from build123d import *

# Parameters (mm, degrees)
SKETCH1_W                = 134
SKETCH1_H                = 134
SKETCH1_W_2              = 20
SKETCH1_H_2              = 13
BOSS_EXTRUDE1_DEPTH      = 1.5
BOSS_EXTRUDE2_DEPTH      = 45
SKETCH2_R                = 1.35
CUT_EXTRUDE1_DEPTH       = 137.5
SKETCH3_W                = 53.4
SKETCH3_H                = 43.5
CUT_EXTRUDE2_DEPTH       = 137.5
SKETCH4_W                = 140
SKETCH4_H                = 5
CUT_EXTRUDE3_DEPTH       = 1.5
SKETCH5_W                = 30
SKETCH5_H                = 43.5
CUT_EXTRUDE4_DEPTH       = 137.5
CUT_EXTRUDE5_DEPTH       = 10
BOSS_EXTRUDE3_DEPTH      = 1.5
BOSS_EXTRUDE4_DEPTH      = 1
BOSS_EXTRUDE5_DEPTH      = 30
BOSS_EXTRUDE5_DEPTH_BACK = 1.5
CUT_EXTRUDE6_DEPTH       = 137.5
SKETCH11_W               = 5
SKETCH11_H               = 40
CUT_EXTRUDE7_DEPTH       = 1.5
BOSS_EXTRUDE6_DEPTH      = 1.5


with BuildPart() as part:
    # Sketch1 → Boss-Extrude1 (new body)
    with BuildSketch(Plane(origin=(0, 0, 0), x_dir=(1, 0, 0), z_dir=(0, 1, 0))):
        Rectangle(SKETCH1_W, SKETCH1_H)
        Rectangle(SKETCH1_W_2, SKETCH1_H_2, mode=Mode.SUBTRACT)
        Polygon((-67, 67), (-67.25, 67.25), (-67.25, -67.25), (67.25, -67.25), (67.25, 67.25), (67, 67), (67, -67), (-67, -67), align=None)
    extrude(amount=BOSS_EXTRUDE1_DEPTH)

    # Sketch1<3> → Boss-Extrude2 (add)
    with BuildSketch(Plane(origin=(0, 0, 0), x_dir=(1, 0, 0), z_dir=(0, 1, 0))):
        Polygon((-67.25, -67.25), (-67.25, 67.25), (-68.75, 68.75), (-68.75, -68.75), (68.75, -68.75), (68.75, 68.75), (67.25, 67.25), (67.25, -67.25), align=None)
    extrude(amount=BOSS_EXTRUDE2_DEPTH)

    # Sketch2 → Cut-Extrude1 (cut)
    with BuildSketch(Plane.ZY.offset(68.75)):
        with Locations((10.85, 42)):
            Circle(SKETCH2_R)
        with Locations((-29.15, 42)):
            Circle(SKETCH2_R)
    extrude(amount=-CUT_EXTRUDE1_DEPTH, mode=Mode.SUBTRACT)

    # Sketch3 → Cut-Extrude2 (cut)
    with BuildSketch(Plane.ZY.offset(68.75)):
        with Locations((40.55, 23.25)):
            Rectangle(SKETCH3_W, SKETCH3_H)
    extrude(amount=-CUT_EXTRUDE2_DEPTH, mode=Mode.SUBTRACT)

    # Sketch4 → Cut-Extrude3 (cut)
    with BuildSketch(Plane.XY.offset(68.75)):
        with Locations((0, 42.5)):
            Rectangle(SKETCH4_W, SKETCH4_H)
    extrude(amount=-CUT_EXTRUDE3_DEPTH, mode=Mode.SUBTRACT)

    # Sketch5 → Cut-Extrude4 (cut)
    with BuildSketch(Plane.ZY.offset(68.75)):
        with Locations((-53.75, 23.25)):
            Rectangle(SKETCH5_W, SKETCH5_H)
    extrude(amount=-CUT_EXTRUDE4_DEPTH, mode=Mode.SUBTRACT)

    # Sketch6 → Cut-Extrude5 (cut)
    with BuildSketch(Plane(origin=(0, 0, 0), x_dir=(-1, 0, 0), z_dir=(0, -1, 0))):
        Polygon((67, 67), (68.75, 67), (68.75, 68.75), align=None)
        Polygon((19.386551984, 67), (68.75, 38.5), (68.75, 67), (67, 67), align=None)
        Polygon((-68.75, 38.5), (-19.386551984, 67), (-67, 67), (-68.75, 67), align=None)
        Polygon((-68.75, 67), (-67, 67), (-68.75, 68.75), align=None)
    extrude(amount=-CUT_EXTRUDE5_DEPTH, mode=Mode.SUBTRACT)


with BuildPart() as body_2:
    # Sketch7 → Boss-Extrude3 (new body)
    with BuildSketch(Plane(origin=(-68.75, 0, 0), x_dir=(0, 0, -1), z_dir=(-1, 0, 0))):
        Polygon((49.15, -63.7), (38.75, -63.7), (38.75, -45), (19.55, -45), (19.55, -63.7), (4.15, -63.7), (4.15, -81.7), (49.15, -81.7), align=None)
    boss_extrude3 = extrude(amount=-BOSS_EXTRUDE3_DEPTH)


with BuildPart() as part_1:
    add(part.part)

    # Mirror6: Boss-Extrude3 across plane
    add(boss_extrude3.mirror(Plane(origin=(0, 0, 0), x_dir=(0, 0, 1), z_dir=(1, 0, 0))))


with BuildPart() as body_2_1:
    add(body_2.part)

    # Combine1: union part
    add(part_1.part)

    # Sketch8 → Boss-Extrude4 (add)
    with BuildSketch(Plane(origin=(0, 1.5, 0), x_dir=(1, 0, 0), z_dir=(0, 1, 0))):
        Polygon((-9.5, 37), (-9.5, 67), (-10.5, 67), (-10.5, 36), (0, 36), (0, 37), align=None)
        Polygon((10.5, 67), (9.5, 67), (9.5, 37), (0, 37), (0, 36), (10.5, 36), align=None)
    extrude(amount=BOSS_EXTRUDE4_DEPTH)

    # Sketch9 → Boss-Extrude5 (add, two sides)
    with BuildSketch(Plane(origin=(0, 1.5, 0), x_dir=(1, 0, 0), z_dir=(0, 1, 0))) as boss_extrude5_sk:
        Polygon((-19.386551984, 67), (-68.25, 38.5), (-68.753822513, 39.363807198), (-19.890374497, 67.863807198), align=None)
        Polygon((19.890374497, 67.863807198), (68.753822513, 39.363807198), (68.25, 38.5), (19.386551984, 67), align=None)
    extrude(amount=BOSS_EXTRUDE5_DEPTH)
    extrude(boss_extrude5_sk.sketch, amount=-BOSS_EXTRUDE5_DEPTH_BACK)

    # Sketch10 → Cut-Extrude6 (cut)
    with BuildSketch(Plane(origin=(68.75, 0, 0), x_dir=(0, 0, -1), z_dir=(1, 0, 0))):
        with BuildLine():
            Line((-13.85, 42), (-13.85, 45))
            Line((-13.85, 45), (-10.85, 45))
            ThreePointArc((-10.85, 45), (-12.971320344, 44.121320344), (-13.85, 42))
        make_face()
    extrude(amount=-CUT_EXTRUDE6_DEPTH, mode=Mode.SUBTRACT)

    # Sketch11 → Cut-Extrude7 (cut)
    with BuildSketch(Plane.XY.offset(68.75)):
        with Locations((66.25, 20)):
            Rectangle(SKETCH11_W, SKETCH11_H)
        with Locations((-66.25, 20)):
            Rectangle(SKETCH11_W, SKETCH11_H)
    extrude(amount=-CUT_EXTRUDE7_DEPTH, mode=Mode.SUBTRACT)


with BuildPart() as body_2_2:
    # Sketch12 → Boss-Extrude6 (new body)
    with BuildSketch(Plane(origin=(68.75, 0, 0), x_dir=(0, 0, -1), z_dir=(1, 0, 0))):
        Polygon((4.15, 63.7), (4.35, 45), (19.55, 45), (19.55, 63.7), align=None)
    extrude(amount=-BOSS_EXTRUDE6_DEPTH)


with BuildPart() as body_3:
    # Mirror8: mirrored copy
    add(body_2_2.part.mirror(Plane(origin=(0, 0, 0), x_dir=(0, 0, 1), z_dir=(1, 0, 0))))


with BuildPart() as body_2_2_1:
    add(body_2_2.part)

    # Combine2: union body 3, body 2
    add(body_3.part)
    add(body_2_1.part)


solid = body_2_2_1.part
Can you work these out from the model? Positions are in its coordinate system, mm. A direction names the side the tool comes from. Give positions to 0.01 mm unless a question says otherwise; leave off trailing zeros. Write each loop counter-clockwise with the first axis right and the second up, starting at its lowest first coordinate (ties: lowest second). Pieces come first, ordered by that corner, then holes. Notation, with made-up numbers: M 44.5,79 L 98.5,79 A31 cw 98.5,113 Z; hole C -15,24 d11. An arc over 180 degrees is marked long. Answer in a Markdown table with one row per item. Add a question column.
Item 1: Imagine slicing it at B-B, the plane y = 48. Write out the boundary of the cut face in (x, z), plus the area to 3 significant figures.
Item 2: Imagine slicing it at C-C, the plane y = 29. Write out the boundary of the cut face in (x, z), plus the area to 3 significant figures.
Item 3: Please list where these lines run through material, in increasing order: L1, parallel to X at y = 35.5, z = -35; L2, parallel to Y at x = -68, z = -29; L3, parallel to Y at x = -67.95, z = 10.85.
Item 4: For pin 1 Ø5 at (x, z) = (-44.5, 24.5) entering from +Y; pin 2 Ø1.1 at (x, y) = (3.5, 2) entering from -Z; pin 3 Ø19 at (y, z) = (25.5, -20) entering from -X, each with a flat end and sliding along its axis, tell me the tip position at first contact or that it passes through.
Item 5: On a 3-axis mill with a long thin cutter (end or side, diameter ignored), from which of +Z, -Z, +X, -X, +Y, -Y can I reach the whole of each face in a straight line? I mean faces 1 (the flat face through (-10, 2.5, -47)), 2 (the flat face through (67.25, 41, -17)), 3 (the flat face through (-1, 1.5, 14)). Say none if no direction works.
Item 6: Imagine slicing it at D-D, the plane x = 38. Write out the boundary of the cut face in (y, z), plus the area to 3 significant figures.
Item 7: We'd pull the mould along Z, two halves only. Please class faces 4 (the flat face through (-43.265, 16.29, -53.073)), 5 (the flat face through (-44.664, 15.97, -53.414)), 6 (the flat face through (0, 1.5, -52)): released by +Z, released by -Z, zero draft, split by the parting line, or undercut.
Item 8: Imagine slicing it at A-A, the plane z = 1. Write out the boundary of the cut face in (x, y).
Evaluation:
| question | item | result |
|---|---|---|
| 1 | outline | M -68.75,-38.75 L -67.25,-38.75 L -67.25,-4.32 L -68.75,-4.32 Z; M 67.25,-38.75 L 68.75,-38.75 L 68.75,-4.32 L 67.25,-4.32 Z |
| 1 | area | 103 mm² |
| 2 | outline | M -68.75,-39.36 L -19.89,-67.86 L -19.39,-67 L -67.82,-38.75 L -67.25,-38.75 L -67.25,13.85 L -68.75,13.85 L -68.75,-38.75 L -68.4,-38.75 Z; M -63.75,67.25 L 63.75,67.25 L 63.75,68.75 L -63.75,68.75 Z; M 19.39,-67 L 19.89,-67.86 L 68.75,-39.36 L 68.4,-38.75 L 68.75,-38.75 L 68.75,13.85 L 67.25,13.85 L 67.25,-38.75 L 67.82,-38.75 Z |
| 2 | area | 462 mm² |
| 3 | L1 | x = -68.75 to -67.25, 67.25 to 68.75 |
| 3 | L2 | y = 0 to 40.66, 43.34 to 81.7 |
| 3 | L3 | y = 0 to 40.65, 43.35 to 45 |
| 4 | pin 1 | stops at y = 1.5 |
| 4 | pin 2 | stops at z = -67 |
| 4 | pin 3 | stops at x = -68.75 |
| 5 | face 1 | -Z, +Y |
| 5 | face 2 | +Z, +Y |
| 5 | face 3 | +Y |
| 6 | outline | M 0,-57.3 L 31.5,-57.3 L 31.5,-56.14 L 1.5,-56.14 L 1.5,67.25 L 40,67.25 L 40,68.75 L 0,68.75 Z |
| 6 | area | 282 mm² |
| 7 | face 4 | undercut |
| 7 | face 5 | released by -Z |
| 7 | face 6 | zero draft |
| 8 | outline | M -68.75,0 L -10,0 L -10,1.5 L -67.25,1.5 L -67.25,45 L -68.75,45 Z; M 10,0 L 68.75,0 L 68.75,45 L 67.25,45 L 67.25,1.5 L 10,1.5 Z |
